Could you check a few things on this model? Use its own coordinates, in mm. A direction names the side the tool comes from. Coordinates: 2 decimals unless noted, no trailing zeros. Order: outer loops, then holes, each group sorted by start corner. A loop starts at its lowest first (then second) coordinate and runs counter-clockwise, first axis right, second up. Notation, with made-up numbers: (-32, 55) - (-28, 55) arc R25 ccw to (-28, 87) - close; hole circle Ø5 at (14.5, -27). An arc over 180 degrees is marked (long way). Answer as a JSON object with one key per item and string values. Group by question number.
(1) We'd pull the mould along Y, two halves only. Please class faces 1 (the flat face through (0, 45, 8)), 2 (the flat face through (0, 200, 0)), 3 (the flat face through (0, 5, 8)), 4 (the cylindrical face through (-1.08, 123.95, 4.88)): pulls with the +Y half, pulls with the -Y half, needs draft (parallel to the pull), parting line crosses it, or undercut.
(2) Please list where these lines run through material, in increasing order: probe 1 along X at (y, z) = (187.5, -0.25); probe 2 along Y at (x, z) = (-2, 6); probe 3 along Z at (x, y) = (0.5, 103).
(3) Which directions (+Z, -Z, +X, -X, +Y, -Y) give clear straight access to the entire face, cutting with the end or side of a thin tool? Please do faces 5 (the cylindrical face through (-7.493, 25.28, -0.33)), 6 (the cylindrical face through (4.57, 47.465, -7.167)), 7 (the flat face through (4, 50, 4)).
(4) Imagine slicing it at C-C, the plane y = 157. Write out the boundary of the cut face in (x, z), and give its area (3 significant figures).
(5) Imagine slicing it at B-B, the plane z = 0. Write out the boundary of the cut face in (x, y).
(6) Imagine slicing it at A-A, the plane x = 0. Write out the boundary of the cut face in (y, z).
(7) Will these pins go through, and if not, where does the flat tip stop? P1, Ø8, axis at x = -6, y = 86, coming from the +Z side; P2, Ø5, axis at y = 100, z = -3, coming from the +X side; P3, Ø6, axis at y = 71.5, z = -4.5, coming from the -X side.
from build123d import *

# Parameters (mm, degrees)
SKETCH1_R           = 8.5
BOSS_EXTRUDE1_DEPTH = 50
SKETCH2_R           = 5
BOSS_EXTRUDE2_DEPTH = 150
SKETCH3_R           = 8.5
SKETCH3_R_2         = 7.5
CUT_EXTRUDE1_DEPTH  = 40


with BuildPart() as part:
    # Sketch1 → Boss-Extrude1 (new body)
    with BuildSketch(Plane(origin=(0, 0, 0), x_dir=(1, 0, 0), z_dir=(0, 1, 0))):
        Circle(SKETCH1_R)
    extrude(amount=BOSS_EXTRUDE1_DEPTH)

    # Sketch2 → Boss-Extrude2 (add)
    with BuildSketch(Plane(origin=(0, 50, 0), x_dir=(1, 0, 0), z_dir=(0, 1, 0))):
        Circle(SKETCH2_R)
    extrude(amount=BOSS_EXTRUDE2_DEPTH)

    # Sketch3 → Cut-Extrude1 (cut)
    with BuildSketch(Plane(origin=(0, 45, 0), x_dir=(1, 0, 0), z_dir=(0, 1, 0))):
        Circle(SKETCH3_R)
        Circle(SKETCH3_R_2, mode=Mode.SUBTRACT)
    extrude(amount=-CUT_EXTRUDE1_DEPTH, mode=Mode.SUBTRACT)


solid = part.part
Result set:
{
 "1": {"face 1": "undercut", "face 2": "pulls with the +Y half", "face 3": "undercut", "face 4": "needs draft"},
 "2": {"probe 1": "x = -4.99 to 4.99", "probe 2": "y = 0 to 50", "probe 3": "z = -4.97 to 4.97"},
 "3": {"face 5": "none", "face 6": "+Y, -Y", "face 7": "+Y"},
 "4": {"outline": "circle Ø10 at (0, 0)", "area": "78.5 mm^2"},
 "5": {"outline": "(-8.5, 0) - (8.5, 0) - (8.5, 5) - (7.5, 5) - (7.5, 45) - (8.5, 45) - (8.5, 50) - (5, 50) - (5, 200) - (-5, 200) - (-5, 50) - (-8.5, 50) - (-8.5, 45) - (-7.5, 45) - (-7.5, 5) - (-8.5, 5) - close"},
 "6": {"outline": "(0, -8.5) - (5, -8.5) - (5, -7.5) - (45, -7.5) - (45, -8.5) - (50, -8.5) - (50, -5) - (200, -5) - (200, 5) - (50, 5) - (50, 8.5) - (45, 8.5) - (45, 7.5) - (5, 7.5) - (5, 8.5) - (0, 8.5) - close"},
 "7": {"P1": "stops at z = 4.58", "P2": "stops at x = 4.97", "P3": "stops at x = -4.77"}
}
